from build123d import *

# Parameters (mm, degrees)
F1_DEPTH = 3
F2_D     = 3
F3_D     = 3
F4_D     = 2.5


with BuildPart() as f1:
    # F0 (on Top) → F1 (new body)
    with BuildSketch(Plane.XY):
        Polygon((-45, -41.623287946), (0, -41.623287946), (0, 28.376712054), (-15, 28.376712054), (-45, 3.376712054), align=None)
    extrude(amount=F1_DEPTH)

    # F2 (through all)
    with Locations(Plane(origin=(0, 0, 0), x_dir=(1, 0, 0), z_dir=(0, 0, -1))):
        with Locations((-22.5, 19.123287946)):
            Hole(F2_D / 2)

    # F3 (through all)
    with Locations(Plane(origin=(0, 0, 0), x_dir=(1, 0, 0), z_dir=(0, 0, -1))):
        with Locations((-18.5292713703, -10.7140789706)):
            Hole(F3_D / 2)

    # F4 (through all)
    with Locations(Plane(origin=(0, 0, 0), x_dir=(1, 0, 0), z_dir=(0, 0, -1))):
        with Locations((-7.5, -20.876712054)):
            Hole(F4_D / 2)


solid = f1.part
The model under review builds one solid part; all positions refer to its coordinate system, in mm. Round coordinates to 2 decimals unless told otherwise and drop trailing zeros. Loops run counter-clockwise (first coordinate to the right, second up) from the corner with the lowest first, then second, coordinate; pieces in that order, holes last. Notation, with made-up numbers: M 64.5,77 L 113.5,77 A32 ccw 113.5,108 Z; hole C 82,24 d11. An arc over 180 degrees is marked long. Answer as CSV lines item,"result". Start each with the question number.
Item 1: Consider section C-C (x = -22.5). Write out the cut boundary in (y, z).
Item 2: Consider section A-A (x = -7.5). Write out the cut boundary in (y, z), then the cut area to 4 significant figures.
Item 3: Consider section D-D (x = -34.5). Write out the cut boundary in (y, z).
Item 4: Mouldability with a two-part tool opening along X and no side actions: class faces 1 (the face through (0, -7, 1)), 2 (the face through (-23, -41.623, 1)), 3 (the face through (-6.58, 20.03, 1.52)) as released by +X, released by -X, zero draft, split by the parting line, or undercut.
Item 5: Consider section B-B (z = 2.5). Write out the cut boundary in (x, y), then the cut area to 3 significant figures.
Item 6: Wall thickness on line 1 (Y direction, x = -22.5, z = 0.8); line 2 (Y direction, x = -7.5, z = 0.85); line 3 (X direction, y = 20, z = 0.7): over which ranges is each line inside the solid? List them lowest first. Write a range as [from, to].
Item 7: Insertion check: P1, Ø2, axis at x = -7.5, y = 20.88, coming from the +Z side. The pin has a flat end and moves straight along its axis. Give the tip position at first contact, or say it passes through.
Answer:
1,outline,"M -41.62,0 L -20.62,0 L -20.62,3 L -41.62,3 Z; M -17.62,0 L 22.13,0 L 22.13,3 L -17.62,3 Z"
2,outline,"M -41.62,0 L 19.63,0 L 19.63,3 L -41.62,3 Z; M 22.13,0 L 28.38,0 L 28.38,3 L 22.13,3 Z"
2,area,"202.5 mm^2"
3,outline,"M -41.62,0 L 12.13,0 L 12.13,3 L -41.62,3 Z"
4,face 1,"released by +X"
4,face 2,"zero draft"
4,face 3,"undercut"
5,outline,"M -45,-41.62 L 0,-41.62 L 0,28.38 L -15,28.38 L -45,3.38 Z; hole C -22.5,-19.12 d3; hole C -18.53,10.71 d3; hole C -7.5,20.88 d2.5"
5,area,"2,760 mm^2"
6,line 1,"y = [-41.62, -20.62], [-17.62, 22.13]"
6,line 2,"y = [-41.62, 19.63], [22.13, 28.38]"
6,line 3,"x = [-25.05, -8.39], [-6.61, 0]"
7,P1,"passes through"
